from build123d import *

# Parameters (mm, degrees)
F0_W     = 393.7
F0_H     = 25.4
F0_W_2   = 25.4
F0_H_2   = 127
F0_W_3   = 304.8
F1_DEPTH = 9.525
F2_W     = 749.3
F2_H     = 20.6375
F2_H_2   = 9.525
F3_DEPTH = 3.175
F4_R     = 3.175
F5_DEPTH = 30.1635


with BuildPart() as f1:
    # F0 (on Front) → F1 (new body)
    with BuildSketch(Plane.XZ):
        with Locations((-132.7033620834, -20.5259278297)):
            Rectangle(F0_W, F0_H)
        with Locations((-342.2533620834, -20.5259278297)):
            Rectangle(F0_W_2, F0_H)
        with Locations((-342.2533620834, -96.7259278297)):
            Rectangle(F0_W_2, F0_H_2)
        with Locations((-507.3533620834, -20.5259278297)):
            Rectangle(F0_W_3, F0_H)
        with Locations((-672.4533620834, -20.5259278297)):
            Rectangle(F0_W_2, F0_H)
        with Locations((-672.4533620834, -96.7259278297)):
            Rectangle(F0_W_2, F0_H_2)
    extrude(amount=F1_DEPTH)

    # F2 (on face) → F3 (join)
    with BuildSketch(Plane.XY.offset(-7.8259278297)):
        with Locations((-310.5033620834, 10.31875)):
            Rectangle(F2_W, F2_H)
        with Locations((-310.5033620834, -4.7625)):
            Rectangle(F2_W, F2_H_2)
        with Locations((-310.5033620834, -19.84375)):
            Rectangle(F2_W, F2_H)
    extrude(amount=F3_DEPTH)

    # F4 (on face) → F5 (cut, through all)
    with BuildSketch(Plane.XZ.offset(9.525)):
        with Locations((-342.2533620834, -96.7259278297)):
            Circle(F4_R)
    extrude(amount=-F5_DEPTH, mode=Mode.SUBTRACT)


solid = f1.part
Verification items for the finished model (mm, model axes). A direction names the side the tool comes from. Give positions to 0.01 mm unless a question says otherwise; leave off trailing zeros. Loops run counter-clockwise (first coordinate to the right, second up) from the corner with the lowest first, then second, coordinate; pieces in that order, holes last.
1) Depth check by flat-ended pin: pin 1 Ø10.5 at (x, y) = (-423.5, -18) entering from -Z; pin 2 Ø10.5 at (x, y) = (-485, -4) entering from -Z; pin 3 Ø5 at (y, z) = (-10, -126) entering from +X; pin 4 Ø12 at (y, z) = (-10, -93) entering from -X. Enter the tip coordinate at first touch or a pass-through.
2) Sectioned sample at B-B, the plane x = -564.5. Enter the section's corners in (y, z) (1 decimal), then the cut area to 3 significant figures.
3) Set-up check for faces 1 (the flat face through (64.147, -5, -15)), 2 (the flat face through (-316, -20, -7.826)), 3 (the flat face through (-368, 0, -33)): record each of +Z, -Z, +X, -X, +Y, -Y from which the full face is reachable in a straight line by a thin tool's end or side.
4) Sectioned sample at D-D, the plane z = -17.5. Enter the section's corners in (x, y) (3 decimals).
5) Thickness scan on line 1 along X through (y, z) = (-9, -54); line 2 along Z through (x, y) = (-188, -28); line 3 along Z through (x, y) = (-188, -3). Record the ranges inside material, lowest first.
6) Sectioned sample at C-C, the plane y = -16. Enter the section's corners in (x, z), then the cut area to 3 significant figures.
7) Sectioned sample at A-A, the plane z = -115. Enter the section's corners in (x, y) (3 decimals), then the cut area to 3 significant figures.
Answers:
1. pin 1: stops at z = -7.83
1. pin 2: stops at z = -33.23
1. pin 3: stops at x = -329.55
1. pin 4: stops at x = -685.15
2. outline: (-30.2, -7.8) - (-9.5, -7.8) - (-9.5, -33.2) - (0, -33.2) - (0, -7.8) - (20.6, -7.8) - (20.6, -4.7) - (-30.2, -4.7) - close
2. area: 403 mm2
3. face 1: +Z, -Z, +X, +Y, -Y
3. face 2: -Z, +X, -X, -Y
3. face 3: -Z, +X, -X, +Y
4. outline: (-685.153, -9.525) - (64.147, -9.525) - (64.147, 0) - (-685.153, 0) - close
5. line 1: x = -685.15 to -659.75, -354.95 to -329.55
5. line 2: z = -7.83 to -4.65
5. line 3: z = -33.23 to -4.65
6. outline: (-685.15, -7.83) - (64.15, -7.83) - (64.15, -4.65) - (-685.15, -4.65) - close
6. area: 2,380 mm2
7. outline: (-685.153, -9.525) - (-659.753, -9.525) - (-659.753, 0) - (-685.153, 0) - close; (-354.953, -9.525) - (-329.553, -9.525) - (-329.553, 0) - (-354.953, 0) - close
7. area: 484 mm2
